from build123d import *

# Parameters (mm, degrees)
SKETCH_1_W          = 20
SKETCH_1_H          = 15
SKETCH_1_W_2        = 18
SKETCH_1_H_2        = 13
EXTRUDE_1_DEPTH     = 550
SKETCH_4_R          = 1.6
CUT_EXTRUDE_1_DEPTH = 551.414616448
SKETCH_5_R          = 2.1
CUT_EXTRUDE_2_DEPTH = 551.414616448
SKETCH_6_R          = 1.6
CUT_EXTRUDE_3_DEPTH = 551.414616448
SKETCH_7_R          = 1.6
CUT_EXTRUDE_4_DEPTH = 551.29537523
SKETCH_8_R          = 1.55
CUT_EXTRUDE_5_DEPTH = 551.414616448


with BuildPart() as part:
    # 草图1 → 拉伸-薄壁1 (new body)
    with BuildSketch(Plane(origin=(0, 0, 0), x_dir=(1, 0, 0), z_dir=(0, 1, 0))):
        Rectangle(SKETCH_1_W, SKETCH_1_H)
        Rectangle(SKETCH_1_W_2, SKETCH_1_H_2, mode=Mode.SUBTRACT)
    extrude(amount=EXTRUDE_1_DEPTH)

    # 草图4 → 切除-拉伸1 (cut, through all)
    with BuildSketch(Plane.ZY.offset(10)):
        with Locations((-3.75, 545)):
            Circle(SKETCH_4_R)
        with Locations(Location((-3.75, 535, 0), (0, 0, 180))):
            Circle(SKETCH_4_R)
        with Locations((3.75, 535)):
            Circle(SKETCH_4_R)
        with Locations(Location((3.75, 545, 0), (0, 0, 180))):
            Circle(SKETCH_4_R)
    extrude(amount=-CUT_EXTRUDE_1_DEPTH, mode=Mode.SUBTRACT)

    # 草图5 → 切除-拉伸2 (cut, through all)
    with BuildSketch(Plane.ZY.offset(10)):
        with Locations((2.5, 512.5)):
            Circle(SKETCH_5_R)
        with Locations((2.5, 477.5)):
            Circle(SKETCH_5_R)
    extrude(amount=-CUT_EXTRUDE_2_DEPTH, mode=Mode.SUBTRACT)

    # 草图6 → 切除-拉伸3 (cut, through all)
    with BuildSketch(Plane(origin=(10, 0, 0), x_dir=(0, 0, -1), z_dir=(1, 0, 0))):
        with Locations((-3.75, 7.5)):
            Circle(SKETCH_6_R)
        with Locations((-3.75, 22.5)):
            Circle(SKETCH_6_R)
        with Locations((3.75, 7.5)):
            Circle(SKETCH_6_R)
        with Locations((3.75, 22.5)):
            Circle(SKETCH_6_R)
        with Locations((-3.75, 92.5)):
            Circle(SKETCH_6_R)
        with Locations((3.75, 92.5)):
            Circle(SKETCH_6_R)
        with Locations((3.75, 77.5)):
            Circle(SKETCH_6_R)
        with Locations((-3.75, 77.5)):
            Circle(SKETCH_6_R)
        with Locations((-3.75, 167.5)):
            Circle(SKETCH_6_R)
        with Locations((-3.75, 182.5)):
            Circle(SKETCH_6_R)
        with Locations((3.75, 167.5)):
            Circle(SKETCH_6_R)
        with Locations((3.75, 182.5)):
            Circle(SKETCH_6_R)
        with Locations((-3.75, 252.5)):
            Circle(SKETCH_6_R)
        with Locations((3.75, 252.5)):
            Circle(SKETCH_6_R)
        with Locations((3.75, 237.5)):
            Circle(SKETCH_6_R)
        with Locations((-3.75, 237.5)):
            Circle(SKETCH_6_R)
        with Locations((-3.75, 327.5)):
            Circle(SKETCH_6_R)
        with Locations((-3.75, 342.5)):
            Circle(SKETCH_6_R)
        with Locations((3.75, 327.5)):
            Circle(SKETCH_6_R)
        with Locations((3.75, 342.5)):
            Circle(SKETCH_6_R)
        with Locations((-3.75, 412.5)):
            Circle(SKETCH_6_R)
        with Locations((3.75, 412.5)):
            Circle(SKETCH_6_R)
        with Locations((3.75, 397.5)):
            Circle(SKETCH_6_R)
        with Locations((-3.75, 397.5)):
            Circle(SKETCH_6_R)
    extrude(amount=-CUT_EXTRUDE_3_DEPTH, mode=Mode.SUBTRACT)

    # 草图7 → 切除-拉伸4 (cut, through all)
    with BuildSketch(Plane(origin=(0, 0, -7.5), x_dir=(-1, 0, 0), z_dir=(0, 0, -1))):
        with Locations((0, 115)):
            Circle(SKETCH_7_R)
        with Locations((0, 135)):
            Circle(SKETCH_7_R)
        with Locations((0, 155)):
            Circle(SKETCH_7_R)
        with Locations((0, 175)):
            Circle(SKETCH_7_R)
        with Locations((0, 195)):
            Circle(SKETCH_7_R)
        with Locations((0, 215)):
            Circle(SKETCH_7_R)
        with Locations((0, 235)):
            Circle(SKETCH_7_R)
        with Locations((0, 255)):
            Circle(SKETCH_7_R)
        with Locations((0, 275)):
            Circle(SKETCH_7_R)
        with Locations((0, 295)):
            Circle(SKETCH_7_R)
        with Locations((0, 315)):
            Circle(SKETCH_7_R)
        with Locations((0, 335)):
            Circle(SKETCH_7_R)
        with Locations((0, 355)):
            Circle(SKETCH_7_R)
        with Locations((0, 375)):
            Circle(SKETCH_7_R)
        with Locations((0, 395)):
            Circle(SKETCH_7_R)
        with Locations((0, 415)):
            Circle(SKETCH_7_R)
        with Locations((0, 435)):
            Circle(SKETCH_7_R)
        with Locations((0, 455)):
            Circle(SKETCH_7_R)
        with Locations((0, 475)):
            Circle(SKETCH_7_R)
        with Locations((0, 495)):
            Circle(SKETCH_7_R)
        with Locations((0, 515)):
            Circle(SKETCH_7_R)
        with Locations((0, 535)):
            Circle(SKETCH_7_R)
    extrude(amount=-CUT_EXTRUDE_4_DEPTH, mode=Mode.SUBTRACT)

    # 草图8 → 切除-拉伸5 (cut, through all)
    with BuildSketch(Plane(origin=(10, 0, 0), x_dir=(0, 0, -1), z_dir=(1, 0, 0))):
        with Locations((5, 377.5)):
            Circle(SKETCH_8_R)
        with Locations(Location((-5, 377.5, 0), (0, 0, 180))):
            Circle(SKETCH_8_R)
        with Locations(Location((5, 362.5, 0), (0, 0, 180))):
            Circle(SKETCH_8_R)
        with Locations((-5, 362.5)):
            Circle(SKETCH_8_R)
        with Locations((5, 57.5)):
            Circle(SKETCH_8_R)
        with Locations(Location((-5, 57.5, 0), (0, 0, 180))):
            Circle(SKETCH_8_R)
        with Locations(Location((5, 42.5, 0), (0, 0, 180))):
            Circle(SKETCH_8_R)
        with Locations((-5, 42.5)):
            Circle(SKETCH_8_R)
    extrude(amount=-CUT_EXTRUDE_5_DEPTH, mode=Mode.SUBTRACT)


solid = part.part
Can you work these out from the model? Positions are in its coordinate system, mm. A direction names the side the tool comes from. Round coordinates to 2 decimals unless told otherwise and drop trailing zeros. Loops run counter-clockwise (first coordinate to the right, second up) from the corner with the lowest first, then second, coordinate; pieces in that order, holes last. Notation, with made-up numbers: (51.5, 36) - (60.5, 36) arc R24 cw to (60.5, 62) - close; hole circle Ø10 at (37, 17.25). An arc over 180 degrees is marked (long way). Answer in a Markdown table with one row per item. Add a question column.
Q1. I want a section at B-B on x = 5. List the corners of the cut face in (y, z) for me.
Q2. Which directions (+Z, -Z, +X, -X, +Y, -Y) give clear straight access to the entire face, cutting with the end or side of a thin tool? Please do faces 1 (the flat face through (0, 463, 6.5)), 2 (the flat face through (-1, 0, 7)).
Q3. I want a section at A-A on y = 71. List the corners of the cut face in (x, z) for me.
Q4. For pin 1 Ø5 at (y, z) = (167.5, 3.75) entering from +X, with a flat end and sliding along its axis, tell me the tip position at first contact or that it passes through.
Q5. I need wall thicknesses on L1, parallel to Z at x = -9.4, y = 252.5; L2, parallel to Z at x = -7, y = 259; L3, parallel to X at y = 329, z = -0.25. Which ranges of each line are inside material? Lowest first, please.
A:
| question | item | result |
|---|---|---|
| 1 | outline | (0, -7.5) - (550, -7.5) - (550, -6.5) - (377.89, -6.5) arc R1.55 cw to (377.11, -6.5) - (362.89, -6.5) arc R1.55 cw to (362.11, -6.5) - (57.89, -6.5) arc R1.55 cw to (57.11, -6.5) - (42.89, -6.5) arc R1.55 cw to (42.11, -6.5) - (0, -6.5) - close; (0, 6.5) - (42.11, 6.5) arc R1.55 cw to (42.89, 6.5) - (57.11, 6.5) arc R1.55 cw to (57.89, 6.5) - (362.11, 6.5) arc R1.55 cw to (362.89, 6.5) - (377.11, 6.5) arc R1.55 cw to (377.89, 6.5) - (550, 6.5) - (550, 7.5) - (0, 7.5) - close |
| 2 | face 1 | +Y, -Y |
| 2 | face 2 | +Z, -Z, +X, -X, -Y |
| 3 | outline | (-10, -7.5) - (10, -7.5) - (10, 7.5) - (-10, 7.5) - close; hole (-9, -6.5) - (9, -6.5) - (9, 6.5) - (-9, 6.5) - close |
| 4 | pin 1 | x = 10 |
| 5 | L1 | -7.5 to -5.35, -2.15 to 2.15, 5.35 to 7.5 |
| 5 | L2 | -7.5 to -6.5, 6.5 to 7.5 |
| 5 | L3 | -10 to -9, 9 to 10 |
